Input: part model. Units: mm. Frame: model coordinates. A direction names the side the tool comes from. Coordinates: 2 decimals unless noted, no trailing zeros. Write each loop counter-clockwise with the first axis right and the second up, starting at its lowest first coordinate (ties: lowest second). Pieces come first, ordered by that corner, then holes. Notation, with made-up numbers: (60.25, -36) - (91.25, -36) arc R25 ccw to (91.25, -5) - close; hole circle Ø4 at (85.25, -27). An arc over 180 degrees is marked (long way). One line per question, with ' | ' between items. Start each with the question number.
1) Reachability of faces 1 (the flat face through (56, 6.3, 8)), 2 (the flat face through (85, 58, 1)), 3 (the flat face through (17.9, 15, 8)) from +Z, -Z, +X, -X, +Y, -Y: full face, straight path, thin tool, end or side. Return the list, or none.
2) Section query C-C on z = 1.5. Give the number of separate pieces and of enclosed holes in the cut face, and give its area (3 significant figures).
3) Section query A-A on x = 40.5. Return loops of the section in (y, z), and give its area (3 significant figures).
4) Line query: line 1 (Y direction, x = 12.5, z = 10.5); line 2 (Y direction, x = 73.5, z = 10.75); line 3 (X direction, y = 17, z = 8). Output: solid intervals per line, ascending.
5) Draft query along X for faces 4 (the cylindrical face through (92.797, 1.141, 6.084)), 5 (the cylindrical face through (1.203, 67.559, 6.084)), 6 (the flat face through (88.5, 34, 8)). Return one class per face: released by +X, released by -X, zero draft, split by the parting line, or undercut.
6) Section query D-D on y = 32. Return loops of the section in (x, z).
7) First-contact query: P1, Ø1.6, axis at x = 1, z = 2, coming from the -Y side; P2, Ø5, axis at x = 14.5, y = 29.5, coming from the +Z side; P3, Ø2, axis at y = 42.5, z = 7.5, coming from the -X side. Flat tips, straight axial feed; report the tip coordinate or a pass-through.
8) Section query B-B on y = 59. Return loops of the section in (x, z), and give its area (4 significant figures).
```python
from build123d import *

# Parameters (mm, degrees)
SKETCH_R     = 1.6
SKETCH_R_2   = 14.075
SKETCH_W     = 58.5
SKETCH_H     = 8.12
PAD_DEPTH    = 12
FILLET_R     = 0.5
FILLET001_R  = 4
SKETCH001_W  = 16.4
SKETCH001_H  = 15.1
POCKET_DEPTH = 9


with BuildPart() as part:
    # Sketch → Pad (new body)
    with BuildSketch(Plane.XY):
        Polygon((0, 0), (94, 0), (94, 68.7), (0, 68.7), (0, 40.2), (1.5, 40.2), (1.5, 7.7), (0, 7.7), align=None)
        with Locations((3.45, 65.25)):
            Circle(SKETCH_R, mode=Mode.SUBTRACT)
        with Locations((90.55, 65.25)):
            Circle(SKETCH_R, mode=Mode.SUBTRACT)
        with Locations((90.55, 3.45)):
            Circle(SKETCH_R, mode=Mode.SUBTRACT)
        with Locations((3.45, 3.45)):
            Circle(SKETCH_R, mode=Mode.SUBTRACT)
        with Locations((59.425, 37.705)):
            Circle(SKETCH_R_2, mode=Mode.SUBTRACT)
        with Locations((47.351152, 25.631152)):
            Circle(SKETCH_R, mode=Mode.SUBTRACT)
        with Locations((71.498848, 25.631152)):
            Circle(SKETCH_R, mode=Mode.SUBTRACT)
        with Locations((71.498848, 49.778848)):
            Circle(SKETCH_R, mode=Mode.SUBTRACT)
        with Locations((47.351152, 49.778848)):
            Circle(SKETCH_R, mode=Mode.SUBTRACT)
        with Locations((55.75, 58.14)):
            Rectangle(SKETCH_W, SKETCH_H, mode=Mode.SUBTRACT)
    extrude(amount=PAD_DEPTH)

    # Fillet
    fillet_edges = [part.edges().sort_by_distance(p)[0] for p in [
        (85, 62.2, 6),
        (85, 54.08, 6),
        (26.5, 54.08, 6),
        (26.5, 62.2, 6),
    ]]
    fillet(fillet_edges, radius=FILLET_R)

    # Fillet001
    fillet001_edges = [part.edges().sort_by_distance(p)[0] for p in [
        (0, 68.7, 6),
        (94, 68.7, 6),
        (94, 0, 6),
        (0, 0, 6),
    ]]
    fillet(fillet001_edges, radius=FILLET001_R)

    # Sketch001 (on Face31 of Fillet001) → Pocket (cut)
    with BuildSketch(Plane.XY.offset(12)):
        with BuildLine():
            Line((26.5, 61.7), (26.5, 57.2))
            Line((26.5, 57.2), (24, 57.2))
            ThreePointArc((24, 57.2), (23.646447, 57.053553), (23.5, 56.7))
            Line((23.5, 56.7), (23.5, 6.8))
            ThreePointArc((23.5, 6.8), (23.646447, 6.446447), (24, 6.3))
            Line((24, 6.3), (88, 6.3))
            ThreePointArc((88, 6.3), (88.353553, 6.446447), (88.5, 6.8))
            Line((88.5, 6.8), (88.5, 61.7))
            ThreePointArc((88.5, 61.7), (88.353553, 62.053553), (88, 62.2))
            Line((88, 62.2), (27, 62.2))
            ThreePointArc((27, 62.2), (26.646447, 62.053553), (26.5, 61.7))
        make_face()
        Polygon((0, 60.5), (22, 60.5), (22, 43.5), (1.5, 43.5), (1.5, 40.7), (17.9, 40.7), (17.9, 25.6), (1.5, 25.6), (1.5, 40.2), (0, 40.2), align=None)
        with Locations((9.7, 15.25)):
            Rectangle(SKETCH001_W, SKETCH001_H)
    extrude(amount=-POCKET_DEPTH, mode=Mode.SUBTRACT)


solid = part.part
```
Answer key:
1) face 1: +Z | face 2: +Z, -Z | face 3: +Z, -X
2) separate pieces: 1 | enclosed holes: 10 | area: 5,230 mm²
3) outline: (0, 0) - (54.08, 0) - (54.08, 3) - (6.3, 3) - (6.3, 12) - (0, 12) - close; (62.2, 0) - (68.7, 0) - (68.7, 12) - (62.2, 12) - close | area: 297 mm²
4) line 1: 0 to 7.7, 22.8 to 25.6, 40.7 to 43.5, 60.5 to 68.7 | line 2: 0 to 6.3, 62.2 to 68.7 | line 3: 17.9 to 23.5, 88.5 to 94
5) face 4: released by +X | face 5: released by -X | face 6: undercut
6) outline: (1.5, 0) - (46.56, 0) - (46.56, 3) - (23.5, 3) - (23.5, 12) - (17.9, 12) - (17.9, 3) - (1.5, 3) - close; (72.29, 0) - (94, 0) - (94, 12) - (88.5, 12) - (88.5, 3) - (72.29, 3) - close
7) P1: y = 0.66 | P2: z = 3 | P3: x = 1.5
8) outline: (0, 0) - (26.5, 0) - (26.5, 12) - (22, 12) - (22, 3) - (0, 3) - close; (85, 0) - (94, 0) - (94, 12) - (88.5, 12) - (88.5, 3) - (85, 3) - close | area: 196.5 mm²
